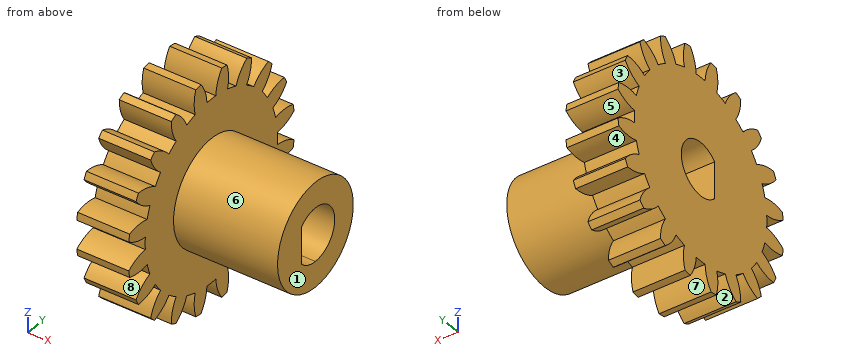
from build123d import *

# Parameters (mm, degrees)
BASPROSKE_W              = 5
BASPROSKE_H              = 11
TOOTHCUT_DEPTH           = 17.340134638
TEETHCUTS_COUNT          = 20
TEETHCUTS_ANGLE          = 342
BORSKE_R                 = 2.5
BORE_DEPTH               = 50.0000508
SKETCH1_R                = 5
BOSS_EXTRUDE2_DEPTH      = 10
BOSS_EXTRUDE2_DEPTH_BACK = 5
CUT_EXTRUDE1_DEPTH       = 22.522623175


with BuildPart() as part:
    # BasProSke → Base-Revolve (revolve)
    with BuildSketch(Plane(origin=(0, 0, 0), x_dir=(1, 0, 0), z_dir=(0, 1, 0)), mode=Mode.PRIVATE) as base_revolve_sk:
        with Locations((2.5, 5.5)):
            Rectangle(BASPROSKE_W, BASPROSKE_H)
    revolve(base_revolve_sk.sketch.rotate(Axis((-10, 0, 0), (1, 0, 0)), 180), axis=Axis((-10, 0, 0), (1, 0, 0)))

    # TooCutSke → ToothCut (cut, through all)
    with BuildSketch(Plane(origin=(0, 0, 0), x_dir=(0, 0, -1), z_dir=(1, 0, 0))):
        with BuildLine():
            ThreePointArc((0.589353609, 8.729127295), (0, 8.749), (-0.589353609, 8.729127295))
            ThreePointArc((-0.589353609, 8.729127295), (-0.82475631, 9.893403384), (-1.391689312, 10.937213814))
            ThreePointArc((-1.391689312, 10.937213814), (0, 11.0254), (1.391689312, 10.937213814))
            ThreePointArc((1.391689312, 10.937213814), (0.82475631, 9.893403384), (0.589353609, 8.729127295))
        make_face()
    toothcut = extrude(amount=TOOTHCUT_DEPTH, mode=Mode.SUBTRACT)

    # TeethCuts: ToothCut ×20 about axis
    teethcuts_axis = Axis((-10, 0, 0), (1, 0, 0))
    for i in range(1, TEETHCUTS_COUNT):
        add(toothcut.rotate(teethcuts_axis, i * TEETHCUTS_ANGLE / (TEETHCUTS_COUNT - 1)), mode=Mode.SUBTRACT)

    # BorSke → Bore (cut, symmetric)
    with BuildSketch(Plane(origin=(0, 0, 0), x_dir=(0, 0, -1), z_dir=(1, 0, 0))):
        with Locations(Location((0, 0, 0), (0, 0, 180))):
            Circle(BORSKE_R)
    extrude(amount=BORE_DEPTH, both=True, mode=Mode.SUBTRACT)

    # Sketch1 → Boss-Extrude2 (add, two sides)
    with BuildSketch(Plane(origin=(5, 0, 0), x_dir=(0, 0, -1), z_dir=(1, 0, 0))) as boss_extrude2_sk:
        Circle(SKETCH1_R)
    extrude(amount=BOSS_EXTRUDE2_DEPTH)
    extrude(boss_extrude2_sk.sketch, amount=-BOSS_EXTRUDE2_DEPTH_BACK)

    # Sketch2 → Cut-Extrude1 (cut, through all)
    with BuildSketch(Plane(origin=(15, 0, 0), x_dir=(0, 0, -1), z_dir=(1, 0, 0))):
        with BuildLine():
            ThreePointArc((2.55, 0), (-1.009950494, 2.341473895), (-1.75, -1.854723699))
            Line((-1.75, -1.854723699), (1.75, -1.854723699))
            ThreePointArc((1.75, -1.854723699), (2.341473895, -1.009950494), (2.55, 0))
        make_face()
    extrude(amount=-CUT_EXTRUDE1_DEPTH, mode=Mode.SUBTRACT)


solid = part.part
CAD build for the part. Positions are in the model's coordinates, mm. Face numbers are marked on the shaded views. A direction names the side the tool comes from. Give positions to 0.01 mm unless a question says otherwise; leave off trailing zeros. Loops run counter-clockwise (first coordinate to the right, second up) from the corner with the lowest first, then second, coordinate; pieces in that order, holes last. Notation, with made-up numbers: M 46.25,-22.5 L 105.25,-22.5 A3 ccw 105.25,-18.5 Z; hole C 86,29 d1. An arc over 180 degrees is marked long. Answer in a Markdown table with one row per item. Add a question column.
Item 1: Drop flat-ended pins along their axis: P1, Ø1, axis at x = 4.5, z = -8, coming from the -Y side; P2, Ø3, axis at x = 3.5, z = 6, coming from the -Y side (3 decimals); P3, Ø3, axis at x = 10.5, z = 4.5, coming from the -Y side. Give the stop position or say it passes through.
Item 2: Tool access for the marked faces 5, 6, 7 and 8: list every direction of +Z, -Z, +X, -X, +Y, -Y with a clear straight run to the whole face (end or side of a thin tool).
Item 3: Band-saw the part on B-B on y = 9.25. Give the cut face in (x, z).
Item 4: Mould opens along Z. For the marked faces 1, 2, 3 and 4 say: +Z half, -Z half, draft (parallel to the pull), parting line (faces both ways), or undercut.
Item 5: Probe probe 1 along Y at (x, z) = (8.25, 0); probe 2 along Y at (x, z) = (3, 6.5); probe 3 along Z at (x, y) = (2.25, -7). List the from-to ranges inside material, lowest first.
Item 6: Band-saw the part on C-C on x = 13.25. Give the cut face in (y, z), then the cut area to 3 significant figures.
Item 7: Band-saw the part on A-A on z = 0. Give the cut face in (x, y), then the cut area to 3 significant figures.
Reply:
| question | item | result |
|---|---|---|
| 1 | P1 | stops at y = -8.02 |
| 1 | P2 | stops at y = -9.955 |
| 1 | P3 | stops at y = -4 |
| 2 | face 5 | +X, -X, +Y |
| 2 | face 6 | +X |
| 2 | face 7 | -Z, +X, -X |
| 2 | face 8 | +X, -X, -Y |
| 3 | outline | M 0,-5.29 L 5,-5.29 L 5,-3.92 L 0,-3.92 Z; M 0,-2.27 L 5,-2.27 L 5,-0.65 L 0,-0.65 Z; M 0,0.65 L 5,0.65 L 5,2.27 L 0,2.27 Z; M 0,3.92 L 5,3.92 L 5,5.29 L 0,5.29 Z |
| 4 | face 1 | draft |
| 4 | face 2 | -Z half |
| 4 | face 3 | undercut |
| 4 | face 4 | undercut |
| 5 | probe 1 | y = -5 to -1.85, 2.55 to 5 |
| 5 | probe 2 | y = -7.53 to 7.53 |
| 5 | probe 3 | z = -7.82 to -5.86, -5.25 to 5.25, 5.86 to 7.82 |
| 6 | outline | C 0,0 d10; hole M -1.85,-1.75 A2.55 ccw long -1.85,1.75 Z |
| 6 | area | 59.8 mm^2 |
| 7 | outline | M 0,-8.75 L 5,-8.75 L 5,-5 L 15,-5 L 15,-1.85 L 0,-1.85 Z; M 0,2.55 L 15,2.55 L 15,5 L 5,5 L 5,8.75 L 0,8.75 Z |
| 7 | area | 121 mm^2 |
